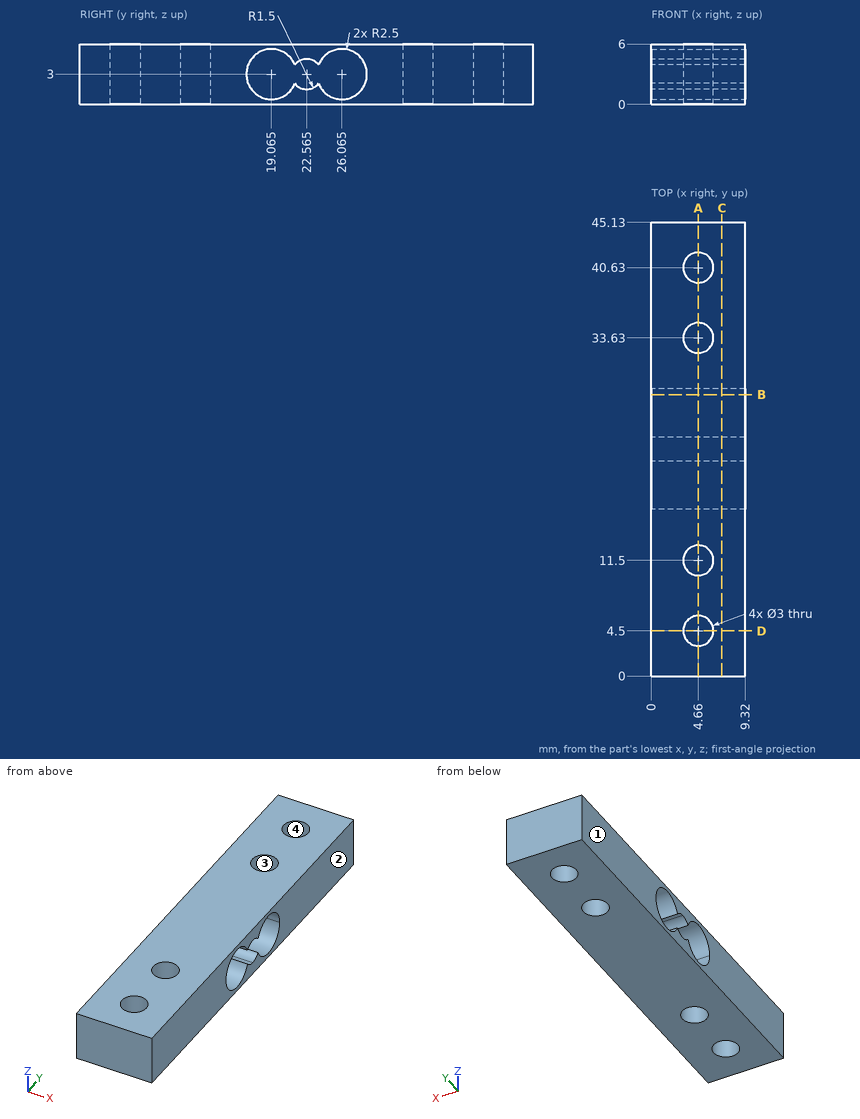
Input: dimensioned drawing with shaded views. Units: mm. Origin: part minimum x, y, z. Round coordinates to 2 decimals unless told otherwise and drop trailing zeros. Loops run counter-clockwise (first coordinate to the right, second up) from the corner with the lowest first, then second, coordinate; pieces in that order, holes last. Notation, with made-up numbers: (73, -2) -> (92, -2) arc R27 ccw to (92, 15) -> close; hole circle Ø10 at (15.5, 62.25). An arc over 180 degrees is marked (long way). Use one line per item in the form item = value. Start each with the question number.
1) Draft query along X for the marked faces 1, 2, 3 and 4. Return one class per face: released by +X, released by -X, zero draft, split by the parting line, or undercut.
2) First-contact query: P1, Ø2.5, axis at x = 4.66, y = 4.5, coming from the +Z side. Flat tip, straight axial feed; report the tip coordinate or a pass-through.
3) Section D-D on y = 4.5. Output: boundary loops of the cut face in (x, z), then the cut area to 3 significant figures.
4) Section B-B on y = 28. Output: boundary loops of the cut face in (x, z), then the cut area to 3 significant figures.
5) Section C-C on x = 7. Output: boundary loops of the cut face in (y, z) (3 decimals), then the cut area to 3 significant figures.
6) Section A-A on x = 4.66. Output: boundary loops of the cut face in (y, z) (3 decimals).
7) Line query: L1, parallel to X at y = 40.5, z = 2.15; L2, parallel to Y at x = 8.75, z = 1.2; L3, parallel to Y at x = 6.75, z = 1.3. Output: solid intervals per line, ascending.
Response:
q1.face_1 = released by -X
q1.face_2 = released by +X
q1.face_3 = undercut
q1.face_4 = undercut
q2.P1 = through
q3.outline = (0, 0) -> (3.16, 0) -> (3.16, 6) -> (0, 6) -> close; (6.16, 0) -> (9.32, 0) -> (9.32, 6) -> (6.16, 6) -> close
q3.area = 37.9 mm^2
q4.outline = (0, 0) -> (9.32, 0) -> (9.32, 1.42) -> (0, 1.42) -> close; (0, 4.58) -> (9.32, 4.58) -> (9.32, 6) -> (0, 6) -> close
q4.area = 26.4 mm^2
q5.outline = (0, 0) -> (45.13, 0) -> (45.13, 6) -> (0, 6) -> close; hole (21.386, 2.072) arc R1.5 ccw to (23.744, 2.072) arc R2.5 ccw (long way) to (23.744, 3.928) arc R1.5 ccw to (21.386, 3.928) arc R2.5 ccw (long way) to start
q5.area = 226 mm^2
q6.outline = (0, 0) -> (3, 0) -> (3, 6) -> (0, 6) -> close; (6, 0) -> (10, 0) -> (10, 6) -> (6, 6) -> close; (13, 0) -> (32.13, 0) -> (32.13, 6) -> (13, 6) -> close; (35.13, 0) -> (39.13, 0) -> (39.13, 6) -> (35.13, 6) -> close; (42.13, 0) -> (45.13, 0) -> (45.13, 6) -> (42.13, 6) -> close; hole (21.386, 2.072) arc R1.5 ccw to (23.744, 2.072) arc R2.5 ccw (long way) to (23.744, 3.928) arc R1.5 ccw to (21.386, 3.928) arc R2.5 ccw (long way) to start
q7.L1 = 0 to 3.17, 6.15 to 9.32
q7.L2 = 0 to 17.33, 20.8 to 24.33, 27.8 to 45.13
q7.L3 = 0 to 17.23, 20.9 to 24.23, 27.9 to 45.13
